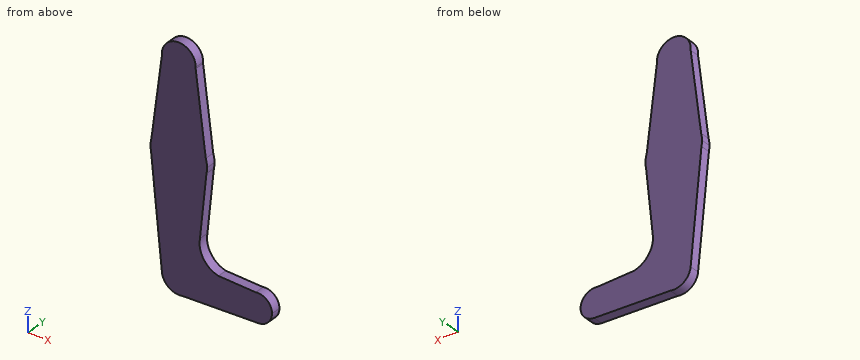
```python
from build123d import *

# Parameters (mm, degrees)
F0_R     = 3.175
F0_R_2   = 1.5875
F1_DEPTH = 5.588


with BuildPart() as f1:
    # F0 (on Front) → F1 (new body)
    with BuildSketch(Plane.XZ):
        with BuildLine():
            ThreePointArc((15.547094004, -3.2099054549), (-0.0454207738, -15.874935022), (-15.5652074351, -3.1208880949))
            Line((-15.5652074351, -3.1208880949), (-9.4824203242, -64.3996275867))
            ThreePointArc((-9.4824203242, -64.3996275867), (-0.4503173391, -53.9856508739), (9.525, -63.5))
            ThreePointArc((9.525, -63.5), (7.3792459071, -69.5226534719), (1.9087575134, -72.8317881328))
            Line((1.9087575134, -72.8317881328), (44.7092226012, -71.4332660294))
            ThreePointArc((44.7092226012, -71.4332660294), (36.5485288978, -64.2554208568), (43.2013451148, -55.6613287333))
            Line((43.2013451148, -55.6613287333), (22.225, -54.7662357154))
            ThreePointArc((22.225, -54.7662357154), (13.8776701671, -48.8669484195), (11.907621819, -38.8370722765))
            Line((11.907621819, -38.8370722765), (15.547094004, -3.2099054549))
        make_face()
        with BuildLine():
            ThreePointArc((15.1641631674, 4.6972098561), (-0.4169440477, 15.8695237062), (-15.3898941796, 3.8944553072))
            ThreePointArc((-15.3898941796, 3.8944553072), (-15.7532567284, 1.9622760889), (-15.875, 0))
            Line((-15.875, 0), (-15.5652074351, -3.1208880949))
            ThreePointArc((-15.5652074351, -3.1208880949), (-0.0454207738, -15.874935022), (15.547094004, -3.2099054549))
            Line((15.547094004, -3.2099054549), (15.875, 0))
            ThreePointArc((15.875, 0), (15.6962848356, 2.3753457345), (15.1641631674, 4.6972098561))
        make_face()
        with Locations((-9.429e-07, -0.0182211279)):
            Circle(F0_R, mode=Mode.SUBTRACT)
        with BuildLine():
            ThreePointArc((9.4824203242, 49.9003724133), (0, 41.275), (-9.4824203242, 49.9003724133))
            Line((-9.4824203242, 49.9003724133), (-15.3898941796, 3.8944553072))
            ThreePointArc((-15.3898941796, 3.8944553072), (-0.4169440477, 15.8695237062), (15.1641631674, 4.6972098561))
            Line((15.1641631674, 4.6972098561), (9.4824203242, 49.9003724133))
        make_face()
        with Locations((-4.310302902, 36.5252)):
            Circle(F0_R_2, mode=Mode.SUBTRACT)
        with BuildLine():
            ThreePointArc((9.525, -63.5), (-0.4503173391, -53.9856508739), (-9.4824203242, -64.3996275867))
            ThreePointArc((-9.4824203242, -64.3996275867), (-5.6670472877, -71.1557298828), (1.9087575134, -72.8317881328))
            ThreePointArc((1.9087575134, -72.8317881328), (7.3792459071, -69.5226534719), (9.525, -63.5))
        make_face()
        with Locations((-0.270415243, -63.8360157609)):
            Circle(F0_R, mode=Mode.SUBTRACT)
        with BuildLine():
            ThreePointArc((9.4824203242, 49.9003724133), (9.5143491261, 50.3496826609), (9.525, 50.8))
            ThreePointArc((9.525, 50.8), (-0.4503173391, 60.3143491261), (-9.4824203242, 49.9003724133))
            ThreePointArc((-9.4824203242, 49.9003724133), (0, 41.275), (9.4824203242, 49.9003724133))
        make_face()
        with Locations((0, 50.8)):
            Circle(F0_R, mode=Mode.SUBTRACT)
        with BuildLine():
            ThreePointArc((43.2013451148, -55.6613287333), (36.5485288978, -64.2554208568), (44.7092226012, -71.4332660294))
            ThreePointArc((44.7092226012, -71.4332660294), (50.1535728122, -69.0202503047), (52.3875, -63.5))
            ThreePointArc((52.3875, -63.5), (49.6023154066, -57.46199104), (43.2013451148, -55.6613287333))
        make_face()
        with Locations((44.3479567766, -64.1064271331)):
            Circle(F0_R, mode=Mode.SUBTRACT)
        with Locations((-0.270415243, -63.8360157609)):
            Circle(F0_R)
        with Locations((0, 50.8)):
            Circle(F0_R)
        with Locations((-9.429e-07, -0.0182211279)):
            Circle(F0_R)
        with Locations((44.3479567766, -64.1064271331)):
            Circle(F0_R)
        with Locations((-4.310302902, 36.5252)):
            Circle(F0_R_2)
        with BuildLine():
            ThreePointArc((15.547094004, -3.2099054549), (15.7928107428, -1.6133052541), (15.875, 0))
            Line((15.875, 0), (15.547094004, -3.2099054549))
        make_face()
        with BuildLine():
            Line((-15.5652074351, -3.1208880949), (-15.875, 0))
            ThreePointArc((-15.875, 0), (-15.7973620113, -1.5681130328), (-15.5652074351, -3.1208880949))
        make_face()
    extrude(amount=F1_DEPTH)


solid = f1.part
```
Work out the finished part from the listing and answer in its coordinate system (mm). Round coordinates to 2 decimals unless told otherwise and drop trailing zeros. Write each loop counter-clockwise with the first axis right and the second up, starting at its lowest first coordinate (ties: lowest second). Pieces come first, ordered by that corner, then holes.
1) Consider probe 1 along X at (y, z) = (-2.5, 50.5); probe 2 along Z at (x, y) = (-0.5, -0.7); probe 3 along X at (y, z) = (-1.85, -49). Determine where each line is inside the solid, lowest interval first.
2) A cutting plane is placed at C-C on z = 33.5. Determine the outline of the cut face in (x, y).
3) A cutting plane is placed at B-B on x = -11. Determine the outline of the cut face in (y, z), and give its area (3 significant figures).
Entries:
1. probe 1: x = -9.52 to 9.52
1. probe 2: z = -73.01 to 60.31
1. probe 3: x = -11.01 to 13.96
2. outline: (-11.59, -5.59) - (11.54, -5.59) - (11.54, 0) - (-11.59, 0) - close
3. outline: (-5.59, -49.11) - (0, -49.11) - (0, 38.08) - (-5.59, 38.08) - close
3. area: 487 mm2
